Autodesk Inventor part; units mm, degrees
ref_plane "YZ Plane" through (0, 0, 0) normal (1, 0, 0) x (0, 1, 0)
ref_plane "XZ Plane" through (0, 0, 0) normal (0, 1, 0) x (-1, 0, 0)
ref_plane "XY Plane" through (0, 0, 0) normal (0, 0, 1) x (1, 0, 0)
sketch "Sketch1" plane through (0, 0, 0) normal (1, 0, 0) x (0, 1, 0)
  line L0 (18.8, 0) -> (-18.8, 0)
  line L1 (-18.8, 0) -> (-18.8, 1.6)
  line L2 (-18.8, 1.6) -> (18.8, 1.6)
  line L3 (18.8, 1.6) -> (18.8, 0)
  line L4 (18.8, 1.6) -> (28.2, -7.7473)
  line L5 (28.2, -7.7473) -> (28.2, -20.4563)
  line L6 (28.2, -20.4563) -> (26.6, -20.4563)
  line L7 (26.6, -20.4563) -> (26.6, -7.7563)
  line L8 (26.6, -7.7563) -> (18.8, 0)
  line L9 (0, 0) -> (0, 1.6)
  line L10 (-18.8, 1.6) -> (-28.2, -7.7473)
  line L11 (-28.2, -7.7473) -> (-28.2, -20.4563)
  line L12 (-26.6, -20.4563) -> (-26.6, -7.7563)
  line L13 (-26.6, -7.7563) -> (-18.8, 0)
  line L14 (-28.2, -20.4563) -> (-26.6, -20.4563)
  dimension "d0" = 1.6
  dimension "d1" = 1.6
  dimension "d3" = 11
  dimension "d4" = 12.7
  dimension "d5" = 56.4
  dimension "d8" = 7.8
extrude "Extrusion1" add sketch "Sketch1" along normal blind 201.549
sketch "Sketch2" plane through (0, 28.2, -7.7473) normal (0, 1, 0) x (1, 0, 0)
  line L0 (0, 12.709) -> (0, 0)
  line L1 (0, 0) -> (201.549, 0)
  line L2 (201.549, 12.709) -> (201.549, 0)
  line L3 (0, 12.709) -> (201.549, 12.709)
  point P0 (0, -7.7473)
  point P1 (5.6, 6.3545)
  point P2 (195.949, 6.3545)
  point P3 (0, 6.3545)
  point P4 (201.549, 6.3545)
  dimension "d11" = 5.6
  dimension "d12" = 5.6
hole "Hole1" at (5.6, 28.2, -14.1018) at (195.949, 28.2, -14.1018) direction (0, -1, 0) diameter 2.459 end up to surface
sketch "Sketch3" plane through (0, -28.2, -20.4563) normal (0, -1, 0) x (1, 0, 0)
  circle A0 centre (195.949, 6.3545) radius 1.2295
  circle A1 centre (5.6, 6.3545) radius 1.2295
  point P0 (0, 20.4563)
hole "Hole2" at (195.949, -28.2, -14.1018) at (5.6, -28.2, -14.1018) direction (0, 1, 0) diameter 2.459 end up to surface
sketch "Sketch4" plane through (0, -18.8, 1.6) normal (0, 0, 1) x (1, 0, 0)
  line L0 (0, 37.6) -> (0, 0)
  line L1 (0, 0) -> (201.549, 0)
  line L2 (201.549, 37.6) -> (201.549, 0)
  line L3 (0, 37.6) -> (201.549, 37.6) construction
  circle A0 centre (100.7745, 18.8) radius 4.0005
  circle A1 centre (100.7745, 27.1312) radius 1.1938
  circle A2 centre (92.4433, 18.8) radius 1.1938
  circle A3 centre (100.7745, 10.4688) radius 1.1938
  circle A4 centre (109.1057, 18.8) radius 1.1938
  line L4 (0, 37.6) -> (201.549, 37.6)
  circle A5 centre (84.1121, 18.8) radius 4.0005
  circle A6 centre (84.1121, 27.1312) radius 1.1938
  circle A7 centre (75.7809, 18.8) radius 1.1938
  circle A8 centre (84.1121, 10.4688) radius 1.1938
  circle A9 centre (92.4433, 18.8) radius 1.1938
  circle A10 centre (117.4369, 18.8) radius 4.0005
  circle A11 centre (117.4369, 27.1312) radius 1.1938
  circle A12 centre (109.1057, 18.8) radius 1.1938
  circle A13 centre (117.4369, 10.4688) radius 1.1938
  circle A14 centre (125.7681, 18.8) radius 1.1938
  point P0 (0, 18.8)
  point P1 (100.7745, 37.6)
  point P2 (201.549, 18.8)
  point P3 (100.7745, 37.6)
  dimension "d27" = 8.001
  dimension "d28" = 8.3312
  dimension "d29" = 2.3876
  dimension "d32" = 360
  dimension "d39" = 8.001
  dimension "d40" = 8.3312
  dimension "d41" = 2.3876
  dimension "d42" = 360
  dimension "d47" = 8.001
  dimension "d48" = 8.3312
  dimension "d49" = 2.3876
  dimension "d50" = 360
  dimension "d53" = 16.6624
  dimension "d54" = 16.6624
extrude "Extrusion2" cut sketch "Sketch4" against normal through all contours A0 | A1 | A2 | A3 | A4 | A5 | A6 | A7 | A8 | A10 | A11 | A13 | A14
equation "\"d54\" = d53"
properties part number "ChassisMainBracket"
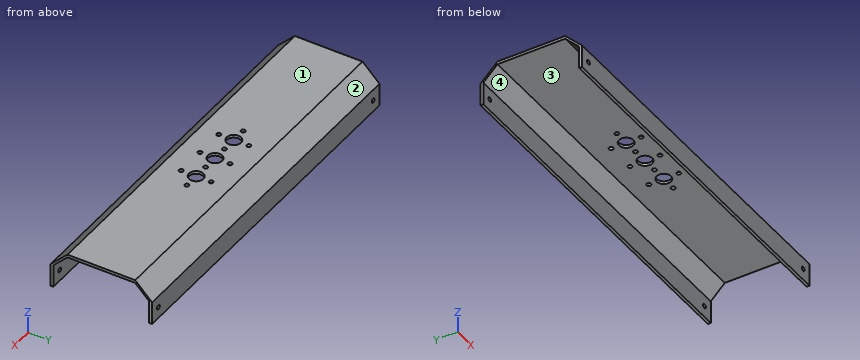
CAD build for the part. Positions are in the model's coordinates, mm. Face numbers are marked on the shaded views. Give positions to 0.01 mm unless a question says otherwise; leave off trailing zeros. Loops run counter-clockwise (first coordinate to the right, second up) from the corner with the lowest first, then second, coordinate; pieces in that order, holes last. Notation, with made-up numbers: (-23.75, 88.5) - (16.25, 88.5) arc R5 ccw to (16.25, 92.5) - close; hole circle Ø5 at (84.5, 72.5). An arc over 180 degrees is marked (long way). Put each result on its own line as item: value.
Q1. Probe line 1 along Y through (x, z) = (123.5, -9.5); line 2 along Z through (x, y) = (163.5, -18); line 3 along Y through (x, z) = (193, -2). List the from-to ranges inside material, lowest first.
Filled in:
line 1: y = -28.2 to -26.6, 26.6 to 28.2
line 2: z = 0 to 1.6
line 3: y = -22.42 to -20.81, 20.81 to 22.42
Q2. Mould opens along Y. For the marked faces 1, 2, 3 and 4 say: pulls with the +Y half, pulls with the -Y half, needs draft (parallel to the pull), parting line crosses it, or undercut.
Filled in:
face 1: needs draft
face 2: pulls with the +Y half
face 3: undercut
face 4: undercut
Q3. Flat gauge pin, fed straight in: pin 1 (19 mm diameter, centred on x = 106, y = -6.5, fed in from -Z). Where does the tip first touch, or does it go through?
Filled in:
pin 1: stops at z = 0
Q4. Slice it at D-D (y = 22). Give the cut face in (x, z).
Filled in:
outline: (0, -3.18) - (201.55, -3.18) - (201.55, -1.58) - (0, -1.58) - close
Q5. Slice it at C-C (y = -15). Give the cut face in (x, z).
Filled in:
outline: (0, 0) - (201.55, 0) - (201.55, 1.6) - (0, 1.6) - close
Q6. Slice it at B-B (x = 137). Give the cut face in (y, z).
Filled in:
outline: (-28.2, -20.46) - (-26.6, -20.46) - (-26.6, -7.76) - (-18.8, 0) - (18.8, 0) - (26.6, -7.76) - (26.6, -20.46) - (28.2, -20.46) - (28.2, -7.75) - (18.8, 1.6) - (-18.8, 1.6) - (-28.2, -7.75) - close
Q7. Slice it at A-A (z = -10). Give the cut face in (x, y).
Filled in:
outline: (0, -28.2) - (201.55, -28.2) - (201.55, -26.6) - (0, -26.6) - close; (0, 26.6) - (201.55, 26.6) - (201.55, 28.2) - (0, 28.2) - close
